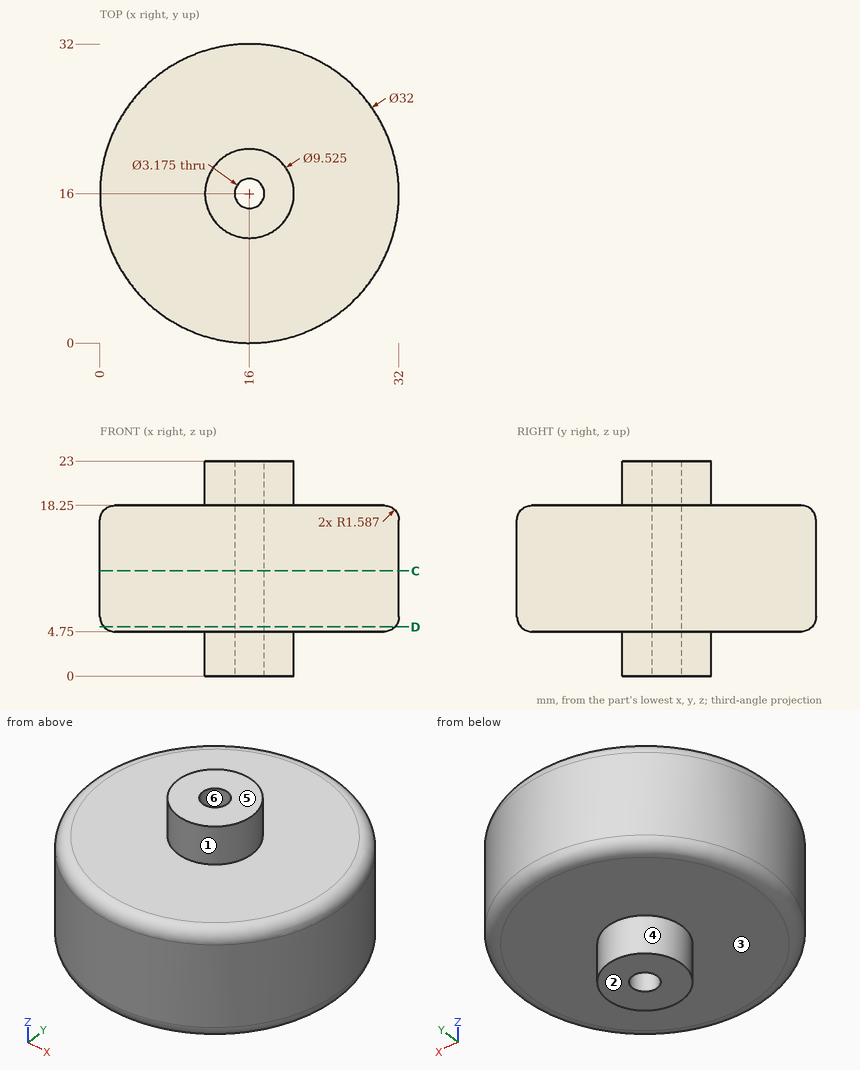
Verification items for this drawing (mm, ordinates from the low corner). A direction names the side the tool comes from. Coordinates: 2 decimals unless noted, no trailing zeros. Order: outer loops, then holes, each group sorted by start corner. A loop starts at its lowest first (then second) coordinate and runs counter-clockwise, first axis right, second up. Notation, with made-up numbers: M 45.25,26.5 L 66.25,26.5 A3 cw 66.25,31.5 Z; hole C 37,-37 d8. An arc over 180 degrees is marked long. Answer as a JSON object with one key per item and string values.
Q1. Cross-section at D-D on z = 5.25. Record the cut outline in (x, y) (1 decimal).
Results are:
{"outline": "C 16,16 d31.1; hole C 16,16 d3.2"}
Q2. Release check for a two-part mould opening along X. For the marked faces 4, 5 and 6 record: released by +X, released by -X, zero draft, split by the parting line, or undercut.
Results are:
{"face 4": "split by the parting line", "face 5": "zero draft", "face 6": "undercut"}
Q3. Cross-section at C-C on z = 11.25. Record the cut outline in (x, y) (1 decimal), and give its area (3 significant figures).
Results are:
{"outline": "C 16,16 d32; hole C 16,16 d3.2", "area": "796 mm²"}
Q4. Tool access check on the marked faces 1, 2 and 3. Record the directions out of +Z, -Z, +X, -X, +Y, -Y that give a thin tool (end or side, any length) a straight path to the whole face; none if there is none.
Results are:
{"face 1": "+Z", "face 2": "-Z, +X, -X, +Y, -Y", "face 3": "-Z"}
Q5. Scan lines: line 1 (Y direction, x = 16, z = 15); line 2 (Z direction, x = 24, y = 8.5); line 3 (Y direction, x = 6, z = 15.75). Record each from-to range of solid material in increasing order.
Results are:
{"line 1": "y = 0 to 14.41, 17.59 to 32", "line 2": "z = 4.75 to 18.25", "line 3": "y = 3.51 to 28.49"}
Q6. Depth check by flat-ended pin: pin 1 Ø1.5 at (x, z) = (15, 16.5) entering from +Y; pin 2 Ø6 at (x, y) = (14, 5) entering from -Z; pin 3 Ø5 at (y, z) = (25, 15.5) entering from -X; pin 4 Ø2.5 at (x, y) = (16, 16) entering from -Z. Enter the tip coordinate at first touch or a pass-through.
Results are:
{"pin 1": "stops at y = 32", "pin 2": "stops at z = 4.75", "pin 3": "stops at x = 1.38", "pin 4": "passes through"}
